Source: CAD feature listing. Evaluate the final solid. Frame: model axes, mm. A direction names the side the tool comes from. Round coordinates to 2 decimals unless told otherwise and drop trailing zeros. Order: outer loops, then holes, each group sorted by start corner. A loop starts at its lowest first (then second) coordinate and runs counter-clockwise, first axis right, second up. Notation, with made-up numbers: (2.5, 26.25) - (27.5, 26.25) arc R7 ccw to (27.5, 39.25) - close; hole circle Ø11 at (87.25, -12.5). An arc over 180 degrees is marked (long way). Return JSON: item names as keys, results as strings. Group by question number.
1) Section D-D, the plane z = 35.5. Return loops of the section in (x, y) (1 decimal), plus the area to 3 significant figures.
2) Ray query, line 1 (Y direction, x = 0, z = 18.5); line 2 (Z direction, x = 0, y = 39.3); line 3 (Y direction, x = -32.5, z = 18). Return the intervals inside material, ascending. Write a range as from..to.
3) Access query for faces 1 (the cylindrical face through (-30.235, 23.183, 24.65)), 2 (the cylindrical face through (0.022, 38.688, 2.465)). Directions: +Z, -Z, +X, -X, +Y, -Y. A direction counts if a zero-diameter tool reaches every point of the face in a straight line with its end or side. Return the directions, or none.
4) Contact query for flat-ended pins moving along their axis: P1, Ø1.8, axis at x = 0, z = 25, coming from the +Y side; P2, Ø3, axis at y = -18, z = 36.5, coming from the -X side (3 decimals); P3, Ø5, axis at x = 18, z = 17, coming from the +Y side; P4, Ø1, axis at y = -28.5, z = 8, coming from the -X side. Output: stop coordinate, or through.
5) Section A-A, the plane y = 0. Return loops of the section in (x, z), plus the area to 3 significant figures.
6) Section B-B, the plane z = 25. Return loops of the section in (x, y) (1 decimal).
7) Mould query, pull axis X, two halves, no side actions, for faces 3 (the cylindrical face through (-0.022, -38.688, 2.465)), 4 (the cylindrical face through (0, 39, 26)), 5 (the flat face through (-14.9, 35.5, 0)), 6 (the cylindrical face through (37.855, -11.921, 24.65)). Classes: pulls with the +X half, pulls with the -X half, needs draft (parallel to the pull), parting line crosses it, or undercut.
8) Section C-C, the plane x = 0. Return loops of the section in (y, z).
Autodesk Inventor part; units mm, degrees
ref_plane "YZ Plane" through (0, 0, 0) normal (1, 0, 0) x (0, 1, 0)
ref_plane "XZ Plane" through (0, 0, 0) normal (0, 1, 0) x (-1, 0, 0)
ref_plane "XY Plane" through (0, 0, 0) normal (0, 0, 1) x (1, 0, 0)
sketch "Sketch1" plane through (0, 0, 0) normal (0, 0, 1) x (1, 0, 0)
  circle A0 centre (0, 0) radius 38.1
  circle A1 centre (0, 0) radius 39.6875
  dimension "d0" = 76.2
  dimension "d1" = 79.375
extrude "Extrusion1" add sketch "Sketch1" along normal blind 50
sketch "Sketch2" plane through (0, 0, 0) normal (1, 0, 0) x (0, 1, 0)
  circle A0 centre (0, 30) radius 1
  line L0 (-39.6875, 0) -> (39.6875, 0)
  point P0 (0, 0)
  dimension "d4" = 2
  dimension "d5" = 30
extrude "Extrusion2" [suppressed]
sketch "Sketch3" plane through (0, 0, 0) normal (0, 1, 0) x (-1, 0, 0)
  circle A0 centre (0, 25) radius 1
  line L0 (-39.6875, 0) -> (39.6875, 0)
  line L1 (39.6875, 50) -> (-39.6875, 50)
  point P0 (0, 0)
  dimension "d8" = 2
  dimension "d12" = 25
extrude "Extrusion3" cut sketch "Sketch3" along normal through all both and the other way through all
sketch "Sketch5" plane through (0, 0, 0) normal (0, 0, -1) x (-1, 0, 0)
  circle A0 centre (0, 39.6875) radius 1
  point P0 (0, 0)
  dimension "d20" = 2
  dimension "d21" = 39.6875
extrude "Extrusion5" cut sketch "Sketch5" against normal blind 5
pattern_circular "Circular Pattern2" count 2 over 360 about axis through (0, 0, 0) along (0, 0, 1) of "Extrusion5"
properties part number "pipe_70mm"
Geometry check:
{
 "1": {"outline": "circle Ø79.4 at (0, 0); hole circle Ø76.2 at (0, 0)", "area": "388 mm2"},
 "2": {"line 1": "-39.69..-38.1, 38.1..39.69", "line 2": "5..24, 26..50", "line 3": "-22.78..-19.88, 19.88..22.78"},
 "3": {"face 1": "+Z, -Z", "face 2": "-Z, +Y"},
 "4": {"P1": "through", "P2": "x = -36.095", "P3": "y = 36.54", "P4": "x = -28.13"},
 "5": {"outline": "(-39.69, 0) - (-38.1, 0) - (-38.1, 50) - (-39.69, 50) - close; (38.1, 0) - (39.69, 0) - (39.69, 50) - (38.1, 50) - close", "area": "159 mm2"},
 "6": {"outline": "(-1, -39.7) - (-1, -38.1) arc R38.1 cw to (-1, 38.1) - (-1, 39.7) arc R39.7 ccw to start; (1, -39.7) arc R39.7 ccw to (1, 39.7) - (1, 38.1) arc R38.1 cw to (1, -38.1) - close"},
 "7": {"face 3": "undercut", "face 4": "undercut", "face 5": "needs draft", "face 6": "parting line crosses it"},
 "8": {"outline": "(-39.69, 5) - (-38.69, 5) - (-38.69, 0) - (-38.1, 0) - (-38.1, 24) - (-39.69, 24) - close; (-39.69, 26) - (-38.1, 26) - (-38.1, 50) - (-39.69, 50) - close; (38.1, 0) - (38.69, 0) - (38.69, 5) - (39.69, 5) - (39.69, 24) - (38.1, 24) - close; (38.1, 26) - (39.69, 26) - (39.69, 50) - (38.1, 50) - close"}
}
